Autodesk Inventor part; units mm, degrees
ref_plane "YZ Plane" through (0, 0, 0) normal (1, 0, 0) x (0, 1, 0)
ref_plane "XZ Plane" through (0, 0, 0) normal (0, 1, 0) x (-1, 0, 0)
ref_plane "XY Plane" through (0, 0, 0) normal (0, 0, 1) x (1, 0, 0)
sketch "S-Base" plane through (0, 0, 0) normal (0, 1, 0) x (-1, 0, 0)
  line L0 (0, 0) -> (11, 0)
  line L1 (11, 0) -> (11, -34.4)
  line L2 (11, -34.4) -> (0, -34.4)
  line L3 (0, -34.4) -> (0, 0)
  circle A0 centre (4, -17.2) radius 3.5
  line L4 (0, -13.9) -> (7.5, -13.9)
  line L5 (7.5, -13.9) -> (7.5, -20.5)
  line L6 (7.5, -20.5) -> (0, -20.5)
  line L7 (0, -20.5) -> (0, -13.9) construction
  line L8 (7.5, -17.2) -> (0, -17.2) construction
  circle A1 centre (4, -17.2) radius 3.75
  point P0 (5.7812, -20.5)
  point P1 (5.7812, -13.9)
  dimension "d1" = 7
  dimension "d0" = 34.4
  dimension "d2" = 17.2
  dimension "d3" = 6.6
  dimension "d4" = 11
  dimension "d5" = 7.5
  dimension "d6" = 0.25
extrude "Ex-Base" add sketch "S-Base" along normal blind 2.5 contours L0 L1 L2 L3 L6 A1 L5 L4 | A1 L4 A0 | L6 A0 A1 | A0 L4 | L4 L5 A1 | L6 A0 | A1 L5 L6
chamfer "Fase1" distance 0.5 angle 45 12 edges at (-11, 1.25, 0) (0, 1.25, 0) (0, 1.25, -34.4) (-11, 1.25, -34.4) (0, 1.25, -20.5) (0, 1.25, -13.9) (-11, 2.5, -17.2) (-11, 0, -17.2) (0, 2.5, -6.95) (0, 0, -6.95) (0, 2.5, -27.45) (0, 0, -27.45)
equation "\"d2\" = 0.5 * d0"
properties part number "ProbeHead_Kabelfixieung_V1"
Geometry: final body of the model. Coordinates: model frame, mm. A direction names the side the tool comes from. Coordinates: 2 decimals unless noted, no trailing zeros. Loops run counter-clockwise (first coordinate to the right, second up) from the corner with the lowest first, then second, coordinate; pieces in that order, holes last. Notation, with made-up numbers: (74, -33.5) - (118, -33.5) arc R18 ccw to (118, -11.5) - close; hole circle Ø6 at (44.25, 78.25). An arc over 180 degrees is marked (long way). Put each result on its own line as item: value. Start each with the question number.
Q1. Line query: line 1 (Z direction, x = -5.75, y = 1); line 2 (Z direction, x = -7.25, y = 1.7); line 3 (X direction, y = 2.1, z = -7). Output: solid intervals per line, ascending.
Q2. Pull-direction query (Z, two-part tool) for faces 1 (the flat face through (-5, 1, 0)), 2 (the flat face through (-3, 1, -20.5)), 3 (the flat face through (0, 1, -28)); classes: released by +Z, released by -Z, zero draft, split by the parting line, or undercut.
Q3. Cut plane C-C, the plane z = -3. Return loops of the section in (x, y).
Q4. Cut plane D-D, the plane z = -17. Return loops of the section in (x, y), and give its area (3 significant figures).
Q5. Cut plane A-A, the plane x = -5. Return loops of the section in (y, z).
Q6. Set-up query: faces 4 (the flat face through (-9, 0, -17)), 5 (the flat face through (-3, 1, -13.9)). Return all of +Z, -Z, +X, -X, +Y, -Y with unobstructed straight access to the full face (end or side cutting, diameter ignored); none if empty.
Q7. Cut plane B-B, the plane y = 1.1. Return loops of the section in (x, z).
Filled sheet:
1. line 1: -34.4 to -20.5, -13.9 to 0
1. line 2: -34.4 to -19.07, -15.33 to 0
1. line 3: -10.9 to -0.1
2. face 1: released by +Z
2. face 2: undercut
2. face 3: zero draft
3. outline: (-11, 0.5) - (-10.5, 0) - (-0.5, 0) - (0, 0.5) - (0, 2) - (-0.5, 2.5) - (-10.5, 2.5) - (-11, 2) - close
4. outline: (-11, 0.5) - (-10.5, 0) - (-7.74, 0) - (-7.74, 2.5) - (-10.5, 2.5) - (-11, 2) - close
4. area: 7.89 mm²
5. outline: (0, -34.4) - (2.5, -34.4) - (2.5, -20.5) - (0, -20.5) - close; (0, -13.9) - (2.5, -13.9) - (2.5, 0) - (0, 0) - close
6. face 4: +Z, -Z, +X, -X, -Y
6. face 5: +X, +Y, -Y
7. outline: (-11, -33.9) - (-10.5, -34.4) - (-0.5, -34.4) - (0, -33.9) - (0, -21) - (-0.5, -20.5) - (-5.78, -20.5) arc R3.75 cw to (-5.78, -13.9) - (-0.5, -13.9) - (0, -13.4) - (0, -0.5) - (-0.5, 0) - (-10.5, 0) - (-11, -0.5) - close
